Autodesk Inventor part; units mm, degrees
ref_plane "YZ Plane" through (0, 0, 0) normal (1, 0, 0) x (0, 1, 0)
ref_plane "XZ Plane" through (0, 0, 0) normal (0, 1, 0) x (-1, 0, 0)
ref_plane "XY Plane" through (0, 0, 0) normal (0, 0, 1) x (1, 0, 0)
sketch "Sketch1" plane through (0, 0, 0) normal (0, 0, 1) x (1, 0, 0)
  line L0 (-7.5, 16.9418) -> (7.5, 16.9418)
  line L1 (7.5, 16.9418) -> (7.5, -16.9418)
  line L2 (7.5, -16.9418) -> (-7.5, -16.9418)
  line L3 (-7.5, -16.9418) -> (-7.5, 16.9418)
  line L4 (-7.5, 16.9418) -> (7.5, -16.9418) construction
  line L5 (7.5, 16.9418) -> (-7.5, -16.9418) construction
  circle A0 centre (0, 9.4418) radius 5.25
  point P0 (0, 0)
  dimension "d0" = 10.5
  dimension "d1" = 7.5
  dimension "d2" = 15
extrude "Extrusion1" add sketch "Sketch1" along normal blind 7.25
fillet "Fillet1" radius 3 2 edges at (7.5, 16.9418, 3.625) (-7.5, 16.9418, 3.625)
sketch "Sketch2" plane through (0, 0, 0) normal (0, 0, -1) x (-1, 0, 0)
  arc A0 (7.5, 13.9418) -> (4.5, 16.9418) centre (4.5, 13.9418) ccw
  line L0 (-4.5, 16.9418) -> (4.5, 16.9418)
  arc A1 (-4.5, 16.9418) -> (-7.5, 13.9418) centre (-4.5, 13.9418) ccw
  line L1 (-7.5, -16.9418) -> (-7.5, 13.9418)
  line L2 (7.5, -16.9418) -> (-7.5, -16.9418)
  line L3 (7.5, 13.9418) -> (7.5, -16.9418)
  circle A2 centre (0, 9.4418) radius 5.25
  circle A3 centre (0, 9.4418) radius 4
  point P0 (0, 0)
  dimension "d6" = 8
extrude "Extrusion2" add sketch "Sketch2" along normal blind 2 contours L3 L2 L1 A1 L0 A0 | A2
sketch "Sketch3" plane through (0, 0, 7.25) normal (0, 0, 1) x (1, 0, 0)
  line L0 (-7.5, -16.9418) -> (7.5, -16.9418)
  line L1 (-7.5, -16.9418) -> (-0.85, -16.9418)
  line L2 (-0.85, -16.9418) -> (-0.85, -3.0582)
  line L3 (-0.85, -3.0582) -> (-7.5, -3.0582)
  line L4 (-7.5, -3.0582) -> (-7.5, -16.9418)
  line L5 (7.5, -3.0582) -> (0.85, -3.0582)
  line L6 (0.85, -3.0582) -> (0.85, -16.9418)
  line L7 (0.85, -16.9418) -> (7.5, -16.9418)
  line L8 (7.5, -16.9418) -> (7.5, -3.0582)
  line L9 (4.5, 16.9418) -> (-4.5, 16.9418)
  point P0 (0, 0)
  point P1 (-0.85, -16.9418)
  dimension "d10" = 0.85
  dimension "d11" = 0.85
  dimension "d12" = 20
extrude "Extrusion3" add sketch "Sketch3" along normal blind 10
fillet "Fillet2" radius 1 4 edges at (7.5, -3.0582, 12.25) (7.5, -16.9418, 7.625) (-7.5, -16.9418, 7.625) (-7.5, -3.0582, 12.25)
properties part number "Solder_aid"
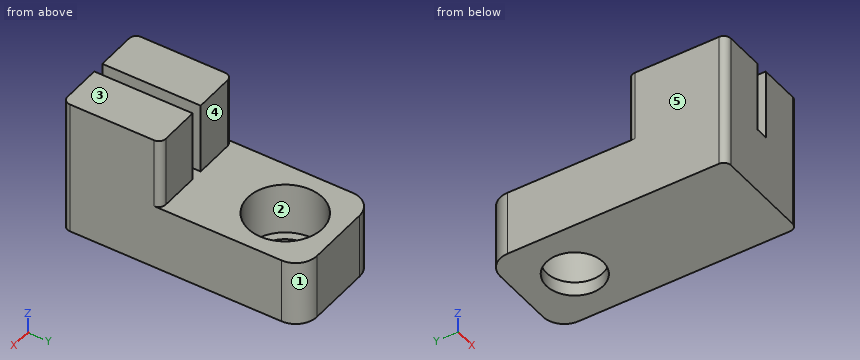
The model under review builds one solid part; all positions refer to its coordinate system, in mm. Face numbers are marked on the shaded views. A direction names the side the tool comes from. Round coordinates to 2 decimals unless told otherwise and drop trailing zeros. Order: outer loops, then holes, each group sorted by start corner. A loop starts at its lowest first (then second) coordinate and runs counter-clockwise, first axis right, second up. Notation, with made-up numbers: M -3.75,79 L 28.25,79 A25 cw 28.25,102 Z; hole C 28.25,21 d9. An arc over 180 degrees is marked long. Use a Markdown table: item, result.
1) Tool access review of the marked faces 4 and 5: name each direction out of +Z, -Z, +X, -X, +Y, -Y from which nothing blocks a thin tool from reaching the whole face with its end or side.
Report:
| item | result |
|---|---|
| face 4 | +Z, +X, -X, +Y |
| face 5 | +Z, -Z, -X, +Y, -Y |
2) Draft analysis for pull direction X (two halves, no side actions). For the marked faces 1, 2 and 3, state which applies: released by +X, released by -X, zero draft, split by the parting line, or undercut.
Report:
| item | result |
|---|---|
| face 1 | released by +X |
| face 2 | undercut |
| face 3 | zero draft |
3) Consider section D-D (z = 0.75). Write out the cut boundary in (x, y), then the cut area to 3 significant figures.
Report:
| item | result |
|---|---|
| outline | M -7.5,-15.94 A1 ccw -6.5,-16.94 L 6.5,-16.94 A1 ccw 7.5,-15.94 L 7.5,13.94 A3 ccw 4.5,16.94 L -4.5,16.94 A3 ccw -7.5,13.94 Z; hole C 0,9.44 d10.5 |
| area | 417 mm^2 |
4) Insertion check: pin 1 (1.7 mm diameter, centred on x = -3.5, z = 14, fed in from +Y); pin 2 (7.5 mm diameter, centred on x = 0, y = -6.5, fed in from +Z). Each pin has a flat end and moves straight along its axis. Give the tip position at first contact, or say it passes through.
Report:
| item | result |
|---|---|
| pin 1 | y = -3.06 |
| pin 2 | z = 17.25 |
5) Wall thickness on line 1 along Y through (x, z) = (0, 2); line 2 along Y through (x, z) = (0, -0.4); line 3 along X through (y, z) = (-4, 10.75): over which ranges is each line inside the solid? List them lowest first. Write a range as [from, to].
Report:
| item | result |
|---|---|
| line 1 | [-16.94, 4.19], [14.69, 16.94] |
| line 2 | [-16.94, 5.44], [13.44, 16.94] |
| line 3 | [-7.5, -0.85], [0.85, 7.5] |
6) Consider section B-B (z = 10.5). Write out the cut boundary in (x, y), then the cut area to 3 significant figures.
Report:
| item | result |
|---|---|
| outline | M -7.5,-15.94 A1 ccw -6.5,-16.94 L -0.85,-16.94 L -0.85,-3.06 L -6.5,-3.06 A1 ccw -7.5,-4.06 Z; M 0.85,-16.94 L 6.5,-16.94 A1 ccw 7.5,-15.94 L 7.5,-4.06 A1 ccw 6.5,-3.06 L 0.85,-3.06 Z |
| area | 184 mm^2 |
7) Consider section A-A (x = 0). Write out the cut boundary in (y, z), then the cut area to 3 significant figures.
Report:
| item | result |
|---|---|
| outline | M -16.94,-2 L 5.44,-2 L 5.44,0 L 4.19,0 L 4.19,7.25 L -16.94,7.25 Z; M 13.44,-2 L 16.94,-2 L 16.94,7.25 L 14.69,7.25 L 14.69,0 L 13.44,0 Z |
| area | 221 mm^2 |
8) Consider section C-C (y = 1). Write out the cut boundary in (x, z), then the cut area to 3 significant figures.
Report:
| item | result |
|---|---|
| outline | M -7.5,-2 L 7.5,-2 L 7.5,7.25 L -7.5,7.25 Z |
| area | 139 mm^2 |
